Can you work these out from the model? Positions are in its coordinate system, mm. A direction names the side the tool comes from. Coordinates: 2 decimals unless noted, no trailing zeros. Write each loop counter-clockwise with the first axis right and the second up, starting at its lowest first coordinate (ties: lowest second). Pieces come first, ordered by that corner, then holes. Notation, with made-up numbers: (33, 64) - (81, 64) arc R26 ccw to (81, 82) - close; hole circle Ø11 at (-9.75, 9). An arc over 180 degrees is marked (long way). Use one line per item in the form item = value. Start each with the question number.
(1) Thinking about a two-plate mould opening in Y: for faces 1 (the face through (177, -2.5, 5)), 2 (the face through (0, 177, 5)), 3 (the face through (362.5, 177, 5)), which applies, pulls with the +Y half, pulls with the -Y half, needs draft (parallel to the pull), parting line crosses it, or undercut?
(2) If I drill on probe 1 along Y at (x, z) = (204.5, 5.75), over which ranges is the centre line in solid material (lowest first)? Write a range as from..to.
(3) If we section it at A-A on y = 250.5: Please give me the cut outline in (x, z).
(4) On a 3-axis mill with a long thin cutter (end or side, diameter ignored), from which of +Z, -Z, +X, -X, +Y, -Y can I reach the whole of each face in a straight line? I mean faces 4 (the face through (177, 362.5, 5)), 5 (the face through (360, 177, 5)). Say none if no direction works.
(5) If we section it at C-C on z = 2.5: Please give me the cut outline in (x, y).
```python
from build123d import *

# Parameters (mm, degrees)
BOX065_W     = 360
BOX065_H     = 360
BOX065_DEPTH = 10
BOX064_W     = 365
BOX064_H     = 365
BOX064_DEPTH = 10


with BuildPart() as cube001:
    # Box065 → Box065 (new body)
    with BuildSketch(Plane(origin=(2.5, 2.5, 0), x_dir=(1, 0, 0), z_dir=(0, 0, 1))):
        with Locations((180, 180)):
            Rectangle(BOX065_W, BOX065_H)
    extrude(amount=BOX065_DEPTH)


with BuildPart() as cut:
    # Box064 → Box064 (new body)
    with BuildSketch(Plane.XY):
        with Locations((182.5, 182.5)):
            Rectangle(BOX064_W, BOX064_H)
    extrude(amount=BOX064_DEPTH)

    # Cut: cut Cube001
    add(cube001.part, mode=Mode.SUBTRACT)


with BuildPart() as cut_1:
    # Cut placement: moved
    add(cut.part.moved(Location((-2.5, -2.5, 0))))


solid = cut_1.part
```
Reported:
q1.face_1 = pulls with the -Y half
q1.face_2 = undercut
q1.face_3 = needs draft
q2.probe_1 = -2.5..0, 360..362.5
q3.outline = (-2.5, 0) - (0, 0) - (0, 10) - (-2.5, 10) - close; (360, 0) - (362.5, 0) - (362.5, 10) - (360, 10) - close
q4.face_4 = +Z, -Z, +X, -X, +Y
q4.face_5 = +Z, -Z
q5.outline = (-2.5, -2.5) - (362.5, -2.5) - (362.5, 362.5) - (-2.5, 362.5) - close; hole (0, 0) - (360, 0) - (360, 360) - (0, 360) - close
